Check sheet for the modelled part. Datum: model origin and axes. Units: mm. Face numbers are marked on the shaded views. Give positions to 0.01 mm unless a question says otherwise; leave off trailing zeros. Write each loop counter-clockwise with the first axis right and the second up, starting at its lowest first coordinate (ties: lowest second). Pieces come first, ordered by that corner, then holes. Notation, with made-up numbers: (-17, 0) -> (7, 0) arc R16 cw to (7, 25) -> close; hole circle Ø8 at (-2, 67). An arc over 180 degrees is marked (long way). Answer as a JSON object with one key per item and string values.
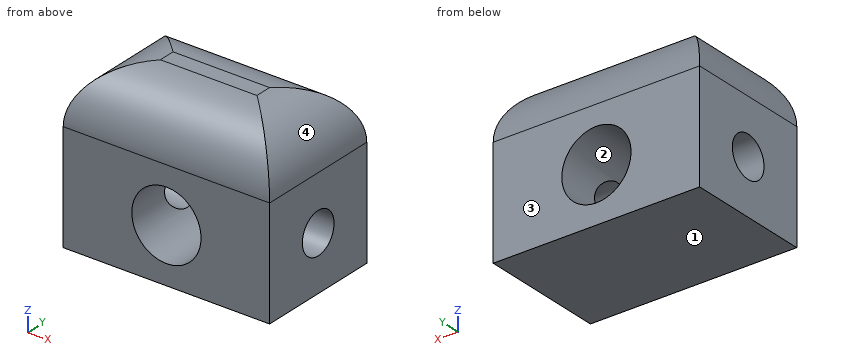
from build123d import *

# Parameters (mm, degrees)
F0_W     = 95.450528
F0_H     = 75.999472
F1_DEPTH = 58.42
F2_R     = 25.4
F3_R     = 16.009617
F4_DEPTH = 58.421
F6_D     = 19.05


with BuildPart() as f1:
    # F0 (on Front) → F1 (new body)
    with BuildSketch(Plane.XZ):
        with Locations((-1.203157, 0.902368)):
            Rectangle(F0_W, F0_H)
    extrude(amount=F1_DEPTH)

    # F2
    f2_edges = [f1.edges().sort_by_distance(p)[0] for p in [
        (-1.203157, -58.42, 38.902104),
        (46.522107, -29.21, 38.902104),
        (-48.928421, -29.21, 38.902104),
        (-1.203157, 0, 38.902104),
    ]]
    fillet(f2_edges, radius=F2_R)

    # F3 (on face) → F4 (cut, through all)
    with BuildSketch(Plane.XZ.offset(58.42)):
        with Locations((-1.203157, -11.797632)):
            Circle(F3_R)
    extrude(amount=-F4_DEPTH, mode=Mode.SUBTRACT)

    # F6 (through all)
    with Locations(Plane.YZ.offset(46.522107)):
        with Locations((-29.21, -11.797632)):
            Hole(F6_D / 2)


solid = f1.part
1. Scan lines: L1, parallel to Z at x = -23, y = -29; L2, parallel to X at y = -44, z = -22.5; L3, parallel to X at y = -31, z = -2. Record each from-to range of solid material in increasing order. Write a range as [from, to].
Determined:
{"L1": "[-37.1, -21.32], [-2.27, 38.9]", "L2": "[-48.93, -13.11], [10.7, 46.52]", "L3": "[-48.93, -13.86], [11.46, 46.52]"}
2. Sectioned sample at B-B, the plane z = -14. Enter the section's corners in (x, y).
Determined:
{"outline": "(-48.93, -58.42) -> (-17.06, -58.42) -> (-17.06, -38.48) -> (-48.93, -38.48) -> close; (-48.93, -19.94) -> (-17.06, -19.94) -> (-17.06, 0) -> (-48.93, 0) -> close; (14.65, -58.42) -> (46.52, -58.42) -> (46.52, -38.48) -> (14.65, -38.48) -> close; (14.65, -19.94) -> (46.52, -19.94) -> (46.52, 0) -> (14.65, 0) -> close"}
3. Sectioned sample at A-A, the plane y = -29.21. Enter the section's corners in (x, z).
Determined:
{"outline": "(-48.93, -37.1) -> (46.52, -37.1) -> (46.52, -21.32) -> (11.66, -21.32) arc R16.01 cw to (-14.07, -21.32) -> (-48.93, -21.32) -> close; (-48.93, -2.27) -> (-14.07, -2.27) arc R16.01 cw to (11.66, -2.27) -> (46.52, -2.27) -> (46.52, 13.5) arc R25.4 ccw to (21.12, 38.9) -> (-23.53, 38.9) arc R25.4 ccw to (-48.93, 13.5) -> close"}
4. Sectioned sample at D-D, the plane x = 26. Enter the section's corners in (y, z) (3 decimals).
Determined:
{"outline": "(-58.42, -37.097) -> (0, -37.097) -> (0, 13.502) arc R25.4 ccw to (-20.522, 38.429) -> (-37.898, 38.429) arc R25.4 ccw to (-58.42, 13.502) -> close; hole circle Ø19.05 at (-29.21, -11.798)"}
5. Go/stop test with flat-tipped pins: P1, Ø1.5, axis at x = 24.5, y = -26, coming from the +Z side; P2, Ø3, axis at y = -36.5, z = 28, coming from the -X side; P3, Ø12, axis at x = -7, y = -46.5, coming from the +Z side. Record where each tip stops, or that it passes through.
Determined:
{"P1": "z = 38.77", "P2": "x = -45.35", "P3": "z = 37.78"}
6. Mould release check, pull along Z, two halves, no side actions. Record for the marked faces 1, 2, 3 and 4: released by +Z, released by -Z, zero draft, split by the parting line, or undercut.
Determined:
{"face 1": "released by -Z", "face 2": "undercut", "face 3": "zero draft", "face 4": "released by +Z"}
7. Sectioned sample at C-C, the plane x = -5. Enter the section's corners in (y, z), plus the area to 3 significant figures.
Determined:
{"outline": "(-58.42, -37.1) -> (0, -37.1) -> (0, -27.35) -> (-58.42, -27.35) -> close; (-58.42, 3.76) -> (0, 3.76) -> (0, 13.5) arc R25.4 ccw to (-25.4, 38.9) -> (-33.02, 38.9) arc R25.4 ccw to (-58.42, 13.5) -> close", "area": "2,350 mm^2"}
